Autodesk Inventor part; units mm, degrees
ref_plane "YZ Plane" through (0, 0, 0) normal (1, 0, 0) x (0, 1, 0)
ref_plane "XZ Plane" through (0, 0, 0) normal (0, 1, 0) x (-1, 0, 0)
ref_plane "XY Plane" through (0, 0, 0) normal (0, 0, 1) x (1, 0, 0)
sketch "Náčrt1" plane through (0, 0, 0) normal (0, 0, 1) x (1, 0, 0)
  line L0 (0, 17.5) -> (0, -17.5)
  line L1 (-28, 0) -> (28, 0)
  line L2 (-20, 12.5) -> (20, 12.5)
  line L3 (20, 12.5) -> (20, -12.5)
  line L4 (20, -12.5) -> (-20, -12.5)
  line L5 (-20, -12.5) -> (-20, 12.5)
  point P0 (0, 0)
  dimension "d0" = 40
  dimension "d1" = 25
extrude "Vysunutí1" add sketch "Náčrt1" along normal mid plane 20
sketch "Náčrt2" plane through (-20, 12.5, -10) normal (0, 1, 0) x (1, 0, 0)
  line L0 (0, 0) -> (40, 0)
  line L1 (0, 0) -> (0, -20)
  line L2 (40, -20) -> (0, -20)
  line L3 (40, 0) -> (40, -20)
  line L4 (-8, -10) -> (48, -10)
  line L5 (20, 4) -> (20, -24)
  line L6 (10, -18.5) -> (30, -18.5)
  line L7 (30, -18.5) -> (30, -1.5)
  line L8 (30, -1.5) -> (10, -1.5)
  line L9 (10, -1.5) -> (10, -18.5)
  point P0 (20, -10)
  dimension "d4" = 17
  dimension "d5" = 20
extrude "Vysunutí2" cut sketch "Náčrt2" against normal blind 15 contours L8 L7 L4 L5 | L5 L4 L9 L8 | L4 L5 L6 L9 | L4 L7 L6 L5
sketch "Náčrt3" plane through (0, 0, 10) normal (0, 0, 1) x (1, 0, 0)
  line L0 (-20, -12.5) -> (20, -12.5)
  line L1 (20, -12.5) -> (20, 12.5)
  line L2 (20, 12.5) -> (-20, 12.5)
  line L3 (-20, 12.5) -> (-20, -12.5)
  line L4 (-10, 12.5) -> (-10, -2.5)
  line L5 (10, 12.5) -> (10, -2.5)
  line L6 (10, -2.5) -> (-10, -2.5)
  line L7 (-28, 0) -> (28, 0)
  line L8 (0, -17.5) -> (0, 17.5)
  line L9 (-10, 12.5) -> (-4.2265, 2.5)
  line L10 (-4.2265, 2.5) -> (4.2265, 2.5)
  line L11 (-20, 12.5) -> (20, 12.5)
  line L12 (4.2265, 2.5) -> (10, 12.5)
  line L13 (-10, 12.5) -> (10, 12.5)
  point P0 (0, 0)
  point P1 (0, 3.8397)
  dimension "d8" = 5
  dimension "d9" = 30
  dimension "d10" = 30
extrude "Vysunutí3" cut sketch "Náčrt3" against normal through all contours L2 L8 L10 L9 | L8 L2 L12 L10
sketch "Náčrt5" plane through (20, -12.5, 10) normal (1, 0, 0) x (0, 0, -1)
  line L0 (20, 25) -> (0, 25)
  line L1 (0, 0) -> (0, 25)
  line L2 (20, 0) -> (0, 0)
  line L3 (20, 25) -> (20, 0)
  line L4 (18.5, 25) -> (18.5, 10)
  line L5 (18.5, 10) -> (1.5, 10)
  line L6 (1.5, 25) -> (1.5, 10)
  line L7 (10, -5) -> (10, 30)
  line L8 (-4, 12.5) -> (24, 12.5)
  line L9 (6.5, 22) -> (13.5, 22)
  line L10 (13.5, 22) -> (13.5, 12)
  line L11 (13.5, 12) -> (6.5, 12)
  line L12 (6.5, 12) -> (6.5, 22)
  line L13 (10, 22) -> (10, 12.5)
  line L14 (13.5, 12.5) -> (10, 12.5)
  line L15 (10, 22) -> (13.5, 22)
  line L16 (13.5, 12.5) -> (13.5, 22)
  dimension "d16" = 7
  dimension "d17" = 10
  dimension "d18" = 3
extrude "Vysunutí4" cut sketch "Náčrt5" against normal through all contours L9 L10 L8 L7 | L7 L8 L12 L9 | L10 L11 L7 L8 | L7 L11 L12 L8
sketch "Náčrt6" plane through (-20, -2.5, -10) normal (0, 1, 0) x (1, 0, 0)
  line L0 (30, -18.5) -> (10, -18.5)
  line L1 (30, -1.5) -> (30, -18.5)
  line L2 (10, -1.5) -> (30, -1.5)
  line L3 (10, -18.5) -> (10, -1.5)
  line L4 (-8, -10) -> (48, -10)
  line L5 (20, 4) -> (20, -24)
  line L6 (13, -6.5) -> (27, -6.5)
  line L7 (27, -6.5) -> (27, -13.5)
  line L8 (27, -13.5) -> (13, -13.5)
  line L9 (13, -13.5) -> (13, -6.5)
  point P0 (20, -10)
  dimension "d21" = 7
  dimension "d22" = 14
  dimension "d23" = 3
extrude "Vysunutí5" cut sketch "Náčrt6" against normal through all contours L8 L9 L4 L5 | L5 L4 L7 L8 | L4 L5 L6 L7 | L4 L9 L6 L5
properties part number "uhelnik_30x30_3D tisk"
Can you work these out from the model? Positions are in its coordinate system, mm. A direction names the side the tool comes from. Coordinates: 2 decimals unless noted, no trailing zeros. Order: outer loops, then holes, each group sorted by start corner. A loop starts at its lowest first (then second) coordinate and runs counter-clockwise, first axis right, second up. Notation, with made-up numbers: (-35.75, 79) - (10.25, 79) arc R22 cw to (10.25, 99) - close; hole circle Ø10 at (55, -27.5). An arc over 180 degrees is marked (long way). Answer as a JSON object with one key per item and string values. Group by question number.
Q1. On a 3-axis mill with a long thin cutter (end or side, diameter ignored), from which of +Z, -Z, +X, -X, +Y, -Y can I reach the whole of each face in a straight line? I mean faces 1 (the face through (10, 5, -4)), 2 (the face through (-15, -0.5, 0)), 3 (the face through (0, -7, -3.5)). Say none if no direction works.
Q2. Imagine slicing it at C-C (z = 8). Please give me the cut outline in (x, y).
Q3. I need wall thicknesses on line 1 (X direction, y = -7.75, z = 1.75); line 2 (Z direction, x = -5.5, y = -1.75); line 3 (X direction, y = 11, z = -8.25). Which ranges of each line are inside material? Lowest first, please. Write a range as from..to.
Q4. We'd pull the mould along Y, two halves only. Please class faces 4 (the face through (15, 5, -3.5)), 5 (the face through (0, 2, 8.5)), 6 (the face through (15, 9.5, 0)), 7 (the face through (0, -12.5, -5)): +Y half, -Y half, draft (parallel to the pull), parting line (faces both ways), or undercut.
Q5. Imagine slicing it at B-B (x = -3.5). Please give me the cut outline in (y, z).
Q6. Will this pin go through, and if not, where does the flat tip stop? P1, Ø0.8, axis at x = -2, z = -9.5, coming from the +Y side.
Q7. Imagine slicing it at D-D (y = 1.5). Please give me the cut outline in (x, z).
Q8. Imagine slicing it at A-A (y = -6.25). Please give me the cut outline in (x, z), and give its area (3 significant figures).
Determined:
{
 "1": {"face 1": "+Y", "face 2": "+X, -X", "face 3": "+Y, -Y"},
 "2": {"outline": "(-20, -12.5) - (20, -12.5) - (20, 12.5) - (10, 12.5) - (10, -2.5) - (-10, -2.5) - (-10, 12.5) - (-20, 12.5) - close"},
 "3": {"line 1": "x = -20..-7, 7..20", "line 2": "z = -10..-8.5, 8.5..10", "line 3": "x = -20..-10, 10..20"},
 "4": {"face 4": "undercut", "face 5": "draft", "face 6": "undercut", "face 7": "-Y half"},
 "5": {"outline": "(-12.5, -10) - (2.5, -10) - (2.5, -8.5) - (-2.5, -8.5) - (-2.5, -3.5) - (-12.5, -3.5) - close; (-12.5, 3.5) - (-2.5, 3.5) - (-2.5, 8.5) - (2.5, 8.5) - (2.5, 10) - (-12.5, 10) - close"},
 "6": {"P1": "stops at y = 2.5"},
 "7": {"outline": "(-20, -10) - (20, -10) - (20, -3.5) - (10, -3.5) - (10, -8.5) - (-10, -8.5) - (-10, -3.5) - (-20, -3.5) - close; (-20, 3.5) - (-10, 3.5) - (-10, 8.5) - (10, 8.5) - (10, 3.5) - (20, 3.5) - (20, 10) - (-20, 10) - close"},
 "8": {"outline": "(-20, -10) - (20, -10) - (20, 10) - (-20, 10) - close; hole (-7, -3.5) - (7, -3.5) - (7, 3.5) - (-7, 3.5) - close", "area": "702 mm2"}
}
